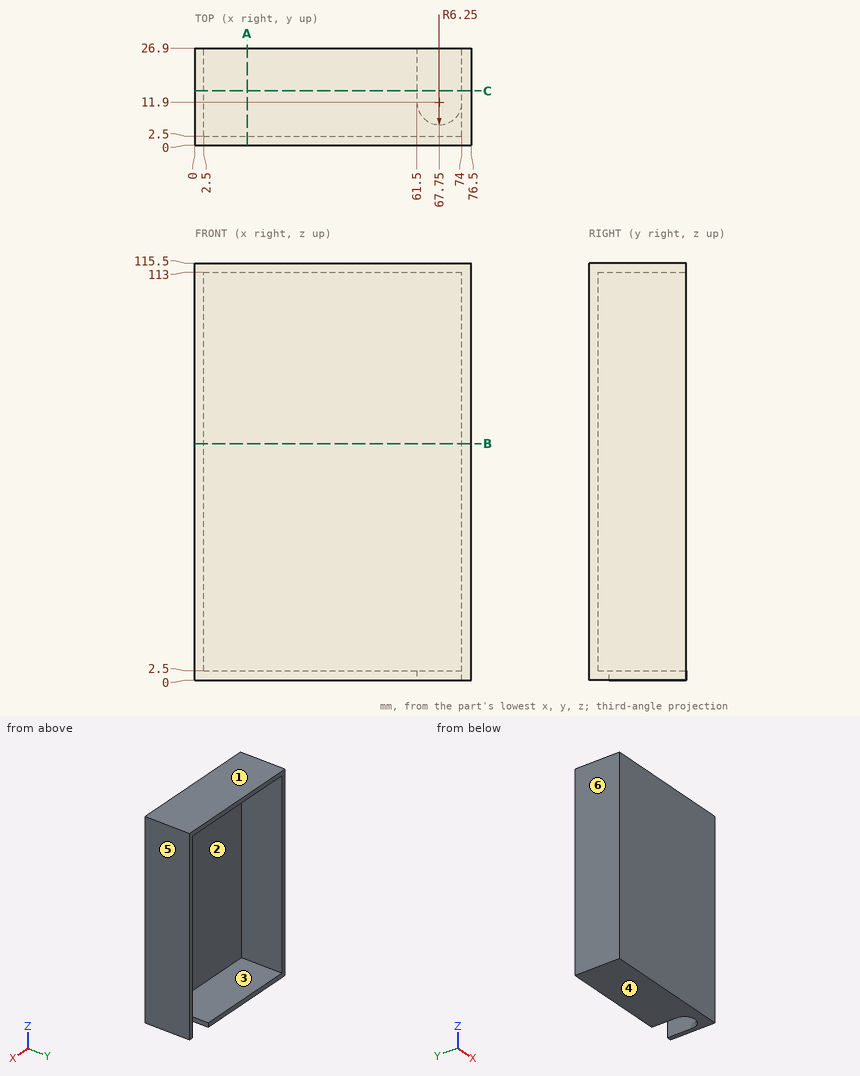
The figure shows three views and two pictorial views of one solid part (mm, origin at its lowest corner). Answer the questions. A direction names the side the tool comes from. Give positions to 0.01 mm unless a question says otherwise; leave off trailing zeros. Order: outer loops, then holes, each group sorted by start corner. A loop starts at its lowest first (then second) coordinate and runs counter-clockwise, first axis right, second up. Notation, with made-up numbers: (65.25, 59) -> (120.25, 59) arc R12 ccw to (120.25, 74) -> close; hole circle Ø6 at (81.25, 80.5). An arc over 180 degrees is marked (long way). Answer as a JSON object with one key per item and string values. Group by question number.
Item 1: The part is cut by section A-A on x = 14.5. Write down the section's boundary in (y, z), and give its area (3 significant figures).
Item 2: Flat-ended cylindrical pins translate along their axes: pin 1 (10 mm diameter, centred on x = 39, y = 12, fed in from -Z); pin 2 (3 mm diameter, centred on x = 33.5, z = 96.5, fed in from +Y). Find the tip coordinate at first contact, or state that the pin passes through.
Item 3: Consider L1, parallel to X at y = 21, z = 20; L2, parallel to Z at x = 34.5, y = 24.5; L3, parallel to Y at x = 11.5, z = 14. Determine where each line is inside the solid, lowest interval first. Write a range as from..to.
Item 4: The part is cut by section C-C on y = 15. Write down the section's boundary in (x, z).
Item 5: Determine the mould class of the marked faces 3, 4, 5 and 6 for opening direction X: pulls with the +X half, pulls with the -X half, needs draft (parallel to the pull), parting line crosses it, or undercut.
Item 6: The part is cut by section B-B on z = 65.5. Write down the section's boundary in (x, y).
Item 7: A tool of negligible diameter and unlimited length cuts with its end or side. For the marked faces 1 and 2, from which of +Z, -Z, +X, -X, +Y, -Y can it reach the whole face along a straight path? Write none if from no direction.
Result set:
{
 "1": {"outline": "(0, 0) -> (26.9, 0) -> (26.9, 2.5) -> (2.5, 2.5) -> (2.5, 113) -> (26.9, 113) -> (26.9, 115.5) -> (0, 115.5) -> close", "area": "411 mm²"},
 "2": {"pin 1": "z = 0", "pin 2": "y = 2.5"},
 "3": {"L1": "0..2.5, 74..76.5", "L2": "0..2.5, 113..115.5", "L3": "0..2.5"},
 "4": {"outline": "(0, 0) -> (61.5, 0) -> (61.5, 2.5) -> (2.5, 2.5) -> (2.5, 113) -> (74, 113) -> (74, 0) -> (76.5, 0) -> (76.5, 115.5) -> (0, 115.5) -> close"},
 "5": {"face 3": "undercut", "face 4": "needs draft", "face 5": "pulls with the +X half", "face 6": "pulls with the -X half"},
 "6": {"outline": "(0, 0) -> (76.5, 0) -> (76.5, 26.9) -> (74, 26.9) -> (74, 2.5) -> (2.5, 2.5) -> (2.5, 26.9) -> (0, 26.9) -> close"},
 "7": {"face 1": "+Z, +X, -X, +Y, -Y", "face 2": "+Y"}
}
